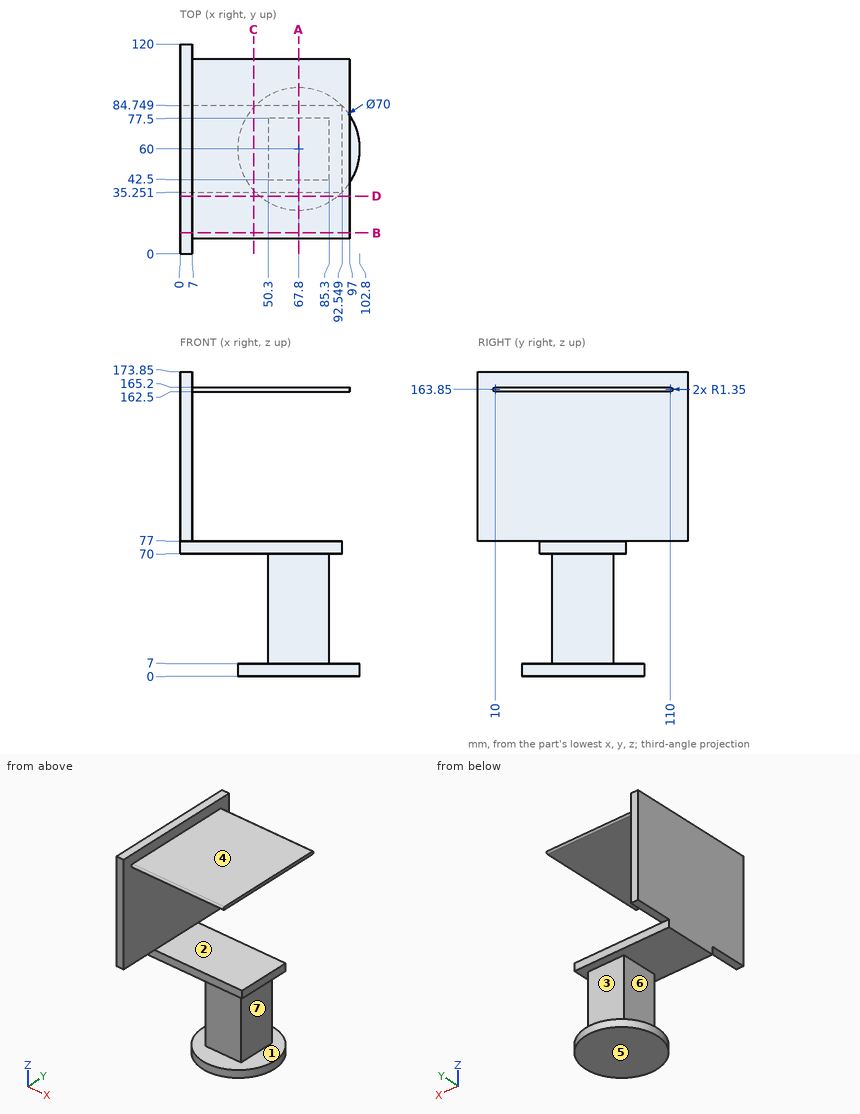
Here's the drawing with two shaded views (mm, measured from the low corner). I have some questions. A direction names the side the tool comes from. Give positions to 0.01 mm unless a question says otherwise; leave off trailing zeros. Loops run counter-clockwise (first coordinate to the right, second up) from the corner with the lowest first, then second, coordinate; pieces in that order, holes last. Notation, with made-up numbers: (68.5, 10) - (120.5, 10) arc R4 ccw to (120.5, 16) - close; hole circle Ø6 at (25, 13.5). An arc over 180 degrees is marked (long way). Answer in a Markdown table with one row per item. Add a question column.
Q1. Please list where these lines run through material, in increasing order: L1, parallel to Z at x = 70, y = 41; L2, parallel to Z at x = 8, y = 50; L3, parallel to Z at x = 71.5, y = 55.5. Write a range as from..to.
Q2. For pin 1 (1 mm diameter, centred on x = 48.5, y = 95, fed in from -Z); pin 2 (15 mm diameter, centred on x = 50.5, y = 62, fed in from +Z); pin 3 (7.5 mm diameter, centred on x = 5, y = 97, fed in from -Z), each with a flat end and sliding along its axis, tell me the tip position at first contact or that it passes through.
Q3. If we section it at C-C (x = 42): List the corners of the cut face in (y, z) for me.
Q4. We'd pull the mould along Z, two halves only. Please class the marked faces 4, 5, 6 and 7: +Z half, -Z half, draft (parallel to the pull), parting line (faces both ways), or undercut.
Q5. Which directions (+Z, -Z, +X, -X, +Y, -Y) give clear straight access to the entire face, cutting with the end or side of a thin tool? Please do the marked faces 1, 2 and 3.
Q6. If we section it at A-A (x = 67.8): List the corners of the cut face in (y, z) for me.
Q7. If we section it at D-D (y = 33): List the corners of the cut face in (x, z) for me.
Q8. If we section it at B-B (y = 12): List the corners of the cut face in (x, z) for me.
The answers:
| question | item | result |
|---|---|---|
| 1 | L1 | z = 0..7, 70..77, 162.5..165.2 |
| 1 | L2 | z = 70..77, 162.5..165.2 |
| 1 | L3 | z = 0..77, 162.5..165.2 |
| 2 | pin 1 | stops at z = 162.5 |
| 2 | pin 2 | stops at z = 165.2 |
| 2 | pin 3 | stops at z = 77 |
| 3 | outline | (10, 162.5) - (110, 162.5) arc R1.35 ccw to (110, 165.2) - (10, 165.2) arc R1.35 ccw to start; (35.25, 70) - (84.75, 70) - (84.75, 77) - (35.25, 77) - close; (36.35, 0) - (83.65, 0) - (83.65, 7) - (36.35, 7) - close |
| 4 | face 4 | +Z half |
| 4 | face 5 | -Z half |
| 4 | face 6 | undercut |
| 4 | face 7 | undercut |
| 5 | face 1 | none |
| 5 | face 2 | +X, +Y, -Y |
| 5 | face 3 | +X, -X, +Y |
| 6 | outline | (10, 162.5) - (110, 162.5) arc R1.35 ccw to (110, 165.2) - (10, 165.2) arc R1.35 ccw to start; (25, 0) - (95, 0) - (95, 7) - (77.5, 7) - (77.5, 70) - (84.75, 70) - (84.75, 77) - (35.25, 77) - (35.25, 70) - (42.5, 70) - (42.5, 7) - (25, 7) - close |
| 7 | outline | (0, 77) - (7, 77) - (7, 162.5) - (97, 162.5) - (97, 165.2) - (7, 165.2) - (7, 173.85) - (0, 173.85) - close; (45.53, 0) - (90.07, 0) - (90.07, 7) - (45.53, 7) - close |
| 8 | outline | (0, 77) - (7, 77) - (7, 162.5) - (97, 162.5) - (97, 165.2) - (7, 165.2) - (7, 173.85) - (0, 173.85) - close |
